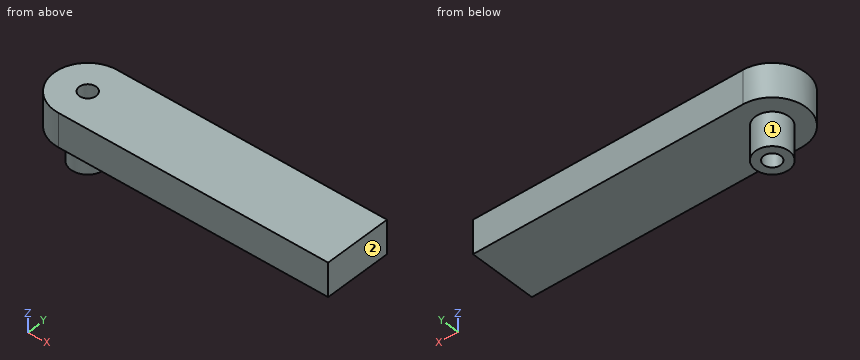
from build123d import *

# Parameters (mm, degrees)
ESTRUSIONE_ESTRUSIONE1_DEPTH = 5
SCHIZZO2_R                   = 2.5
ESTRUSIONE_ESTRUSIONE2_DEPTH = 5
SCHIZZO3_R                   = 1.25
TAGLIO_ESTRUSIONE1_DEPTH     = 11


with BuildPart() as part:
    # Schizzo1 → Estrusione-Estrusione1 (new body)
    with BuildSketch(Plane.XY):
        with BuildLine():
            Line((20, 4.503546099), (-20, 4.503546099))
            ThreePointArc((-20, 4.503546099), (-25, -0.496453901), (-20, -5.496453901))
            Line((-20, -5.496453901), (20, -5.496453901))
            Line((20, -5.496453901), (20, 4.503546099))
        make_face()
    extrude(amount=ESTRUSIONE_ESTRUSIONE1_DEPTH)

    # Schizzo2 → Estrusione-Estrusione2 (add)
    with BuildSketch(Plane(origin=(0, 0, 0), x_dir=(-1, 0, 0), z_dir=(0, 0, -1))):
        with Locations((20, -0.496453901)):
            Circle(SCHIZZO2_R)
    extrude(amount=ESTRUSIONE_ESTRUSIONE2_DEPTH)

    # Schizzo3 → Taglio-Estrusione1 (cut, through all)
    with BuildSketch(Plane(origin=(0, 0, -5), x_dir=(-1, 0, 0), z_dir=(0, 0, -1))):
        with Locations((20, -0.496453901)):
            Circle(SCHIZZO3_R)
    extrude(amount=-TAGLIO_ESTRUSIONE1_DEPTH, mode=Mode.SUBTRACT)


solid = part.part
The model under review builds one solid part; all positions refer to its coordinate system, in mm. Face numbers are marked on the shaded views. A direction names the side the tool comes from. Coordinates: 2 decimals unless noted, no trailing zeros. Write each loop counter-clockwise with the first axis right and the second up, starting at its lowest first coordinate (ties: lowest second). Pieces come first, ordered by that corner, then holes. Notation, with made-up numbers: (-3, 31) - (29, 31) arc R21 cw to (29, 67) - close; hole circle Ø9 at (-18, 82.25). An arc over 180 degrees is marked (long way). Answer as CSV lines item,"result".
(1) Tool access review of the marked faces 1 and 2: name each direction out of +Z, -Z, +X, -X, +Y, -Y from which nothing blocks a thin tool from reaching the whole face with its end or side.
Data:
face 1,"-Z"
face 2,"+Z, -Z, +X, +Y, -Y"
(2) For line 1 along Y through (x, z) = (-20, 1.5); line 2 along X through (y, z) = (-0.5, -0.5); line 3 along Y through (x, z) = (-20, -1.5), list the stretches that pass through material, from the lowest coordinate up. Write a range as [from, to].
Data:
line 1,"y = [-5.5, -1.75], [0.75, 4.5]"
line 2,"x = [-22.5, -21.25], [-18.75, -17.5]"
line 3,"y = [-3, -1.75], [0.75, 2]"
(3) We need section B-B (z = 1). Give the boundary of the cut face in (x, y).
Data:
outline,"(-20, -5.5) - (20, -5.5) - (20, 4.5) - (-20, 4.5) arc R5 ccw to start; hole circle Ø2.5 at (-20, -0.5)"
(4) We need section C-C (x = -18). Give the boundary of the cut face in (y, z), plus the area to 3 significant figures.
Data:
outline,"(-5.5, 0) - (-2, 0) - (-2, -5) - (1, -5) - (1, 0) - (4.5, 0) - (4.5, 5) - (-5.5, 5) - close"
area,"65.0 mm2"
(5) Clearance check with flat-ended pins moving along their axes: pin 1 Ø5 at (y, z) = (0.5, -4) entering from -X; pin 2 Ø1.5 at (x, y) = (-10.5, -1) entering from -Z; pin 3 Ø4 at (y, z) = (3, -1) entering from +X; pin 4 Ø1.5 at (x, y) = (-20, -0.5) entering from +Z. State where each tip first meets the part, or that it passes through.
Data:
pin 1,"stops at x = -22.5"
pin 2,"stops at z = 0"
pin 3,"stops at x = 20"
pin 4,"passes through"
(6) We need section A-A (x = 9). Give the boundary of the cut face in (y, z), plus the area to 3 significant figures.
Data:
outline,"(-5.5, 0) - (4.5, 0) - (4.5, 5) - (-5.5, 5) - close"
area,"50.0 mm2"
(7) We need section D-D (z = -3.5). Give the boundary of the cut face in (x, y).
Data:
outline,"circle Ø5 at (-20, -0.5); hole circle Ø2.5 at (-20, -0.5)"
